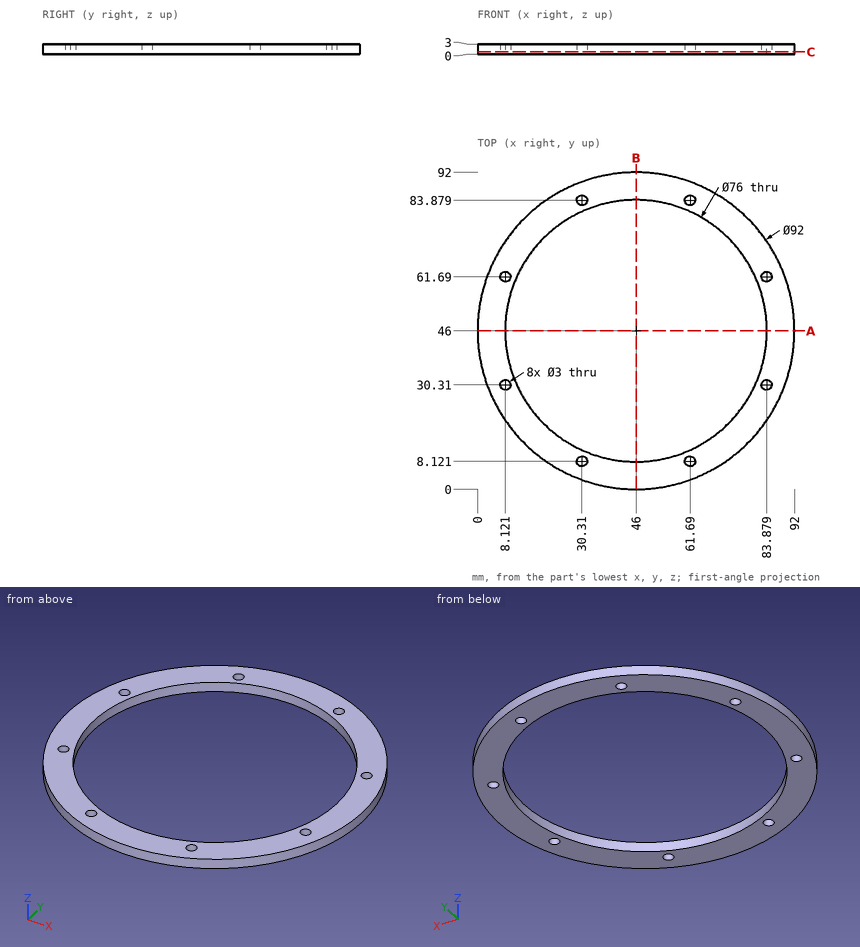
Geometry: see drawing. Coordinates: mm, zero at the bounding-box minimum. Coordinates: 2 decimals unless noted, no trailing zeros. Loops run counter-clockwise (first coordinate to the right, second up) from the corner with the lowest first, then second, coordinate; pieces in that order, holes last. Notation, with made-up numbers: (51.25, 25) - (97.25, 25) arc R8 cw to (97.25, 37) - close; hole circle Ø7 at (87.25, 5.25). An arc over 180 degrees is marked (long way). Return JSON: item names as keys, results as strings.
Q1. Section C-C, the plane z = 0.7. Give the number of separate pieces and of enclosed holes in the cut face, plus the area to 3 significant figures.
Results:
{"separate pieces": "1", "enclosed holes": "9", "area": "2,050 mm2"}
Q2. Contact query for flat-ended pins moving along their axis: P1, Ø2.5, axis at x = 8.12, y = 30.31, coming from the +Z side; P2, Ø3.5, axis at x = 61.69, y = 83.88, coming from the -Z side; P3, Ø1.5, axis at y = 70.5, z = 2, coming from the -X side. Output: stop coordinate, or through.
Results:
{"P1": "through", "P2": "z = 0", "P3": "x = 6.61"}
Q3. Material intervals for line 1 along Y through (x, z) = (29.5, 1.6); line 2 along X through (y, z) = (30.5, 1.1) (3 decimals); line 3 along Y through (x, z) = (46, 1.8), sorted ascending.
Results:
{"line 1": "3.06 to 6.86, 9.38 to 11.77, 80.23 to 82.62, 85.14 to 88.94", "line 2": "2.69 to 6.633, 9.609 to 11.305, 80.695 to 82.391, 85.367 to 89.31", "line 3": "0 to 8, 84 to 92"}
Q4. Section A-A, the plane y = 46. Return loops of the section in (x, z).
Results:
{"outline": "(0, 0) - (8, 0) - (8, 3) - (0, 3) - close; (84, 0) - (92, 0) - (92, 3) - (84, 3) - close"}
